```python
from build123d import *

# Parameters (mm, degrees)
SKETCH2_R           = 12
SKETCH2_R_2         = 2.2
SKETCH2_R_3         = 2.7
BOSS_EXTRUDE1_DEPTH = 5
SKETCH2_4_R         = 4.5
BOSS_EXTRUDE2_DEPTH = 2
FILLET1_R           = 5
FILLET2_R           = 5
SKETCH3_R           = 4.7
SKETCH3_R_2         = 2.7
BOSS_EXTRUDE3_DEPTH = 1
FILLET4_R           = 1
SKETCH4_R           = 6.5
SKETCH4_R_2         = 4.5
BOSS_EXTRUDE5_DEPTH = 1
BOSS_EXTRUDE6_DEPTH = 3


with BuildPart() as part:
    # Sketch2 → Boss-Extrude1 (new body)
    with BuildSketch(Plane(origin=(0, 0, 0), x_dir=(1, 0, 0), z_dir=(0, 1, 0))):
        with BuildLine():
            Line((-32.658907628, 22.065310299), (-15.027926619, -31.62041432))
            Line((-15.027926619, -31.62041432), (-3.044319626, -14.687822099))
            ThreePointArc((-3.044319626, -14.687822099), (14.508216797, 3.809415358), (-9.86730521, 11.297623108))
            Line((-9.86730521, 11.297623108), (-32.658907628, 22.065310299))
        make_face()
        with Locations(Location((0, 0, 0), (0, 0, 270))):
            Circle(SKETCH2_R, mode=Mode.SUBTRACT)
        with Locations(Location((-13.044155697, -18.431125905, 0), (0, 0, 270))):
            Circle(SKETCH2_R_2, mode=Mode.SUBTRACT)
        with Locations(Location((-22.604306415, 10.679200882, 0), (0, 0, 270))):
            Circle(SKETCH2_R_3, mode=Mode.SUBTRACT)
    extrude(amount=BOSS_EXTRUDE1_DEPTH)

    # Sketch2<4> → Boss-Extrude2 (add)
    # profile 1 of 2: a face of its own
    with BuildSketch(Plane(origin=(0, 0, 0), x_dir=(1, 0, 0), z_dir=(0, 1, 0))):
        with BuildLine():
            Line((9.028311423, 2.370559296), (-1.105938309, -11.948928841))
            ThreePointArc((-1.105938309, -11.948928841), (8.084823445, -8.867673306), (12, 0))
            ThreePointArc((12, 0), (5.567714695, 10.630171827), (-6.833425512, 9.864293983))
            Line((-6.833425512, 9.864293983), (9.028311423, 2.370559296))
        make_face()
    # profile 2 of 2: a face of its own
    with BuildSketch(Plane(origin=(0, 0, 0), x_dir=(1, 0, 0), z_dir=(0, 1, 0))):
        with BuildLine():
            ThreePointArc((-6.833425512, 9.864293983), (-11.606573438, -3.047532287), (-1.105938309, -11.948928841))
            Line((-1.105938309, -11.948928841), (9.028311423, 2.370559296))
            Line((9.028311423, 2.370559296), (-6.833425512, 9.864293983))
        make_face()
        with Locations(Location((0, 0, 0), (0, 0, 270))):
            Circle(SKETCH2_4_R, mode=Mode.SUBTRACT)
    extrude(amount=BOSS_EXTRUDE2_DEPTH)

    # Fillet1
    fillet1_edges = [part.edges().sort_by_distance(p)[0] for p in [
        (-15.027926619, 2.5, 31.62041432),
        (-32.658907628, 2.5, -22.065310299),
    ]]
    fillet(fillet1_edges, radius=FILLET1_R)

    # Fillet2
    fillet2_edges = [part.edges().sort_by_distance(p)[0] for p in [
        (-9.86730521, 2.5, -11.297623108),
        (-3.044319626, 2.5, 14.687822099),
    ]]
    fillet(fillet2_edges, radius=FILLET2_R)

    # Sketch3 → Boss-Extrude3 (add)
    with BuildSketch(Plane(origin=(0, 5, 0), x_dir=(1, 0, 0), z_dir=(0, 1, 0))):
        with Locations(Location((-22.604306415, 10.679200882, 0), (0, 0, 270))):
            Circle(SKETCH3_R)
        with Locations(Location((-22.604306415, 10.679200882, 0), (0, 0, 270))):
            Circle(SKETCH3_R_2, mode=Mode.SUBTRACT)
    extrude(amount=BOSS_EXTRUDE3_DEPTH)

    # Fillet4
    fillet4_edges = [part.edges().sort_by_distance(p)[0] for p in [
        (-22.604306415, 5, -15.379200882),
    ]]
    fillet(fillet4_edges, radius=FILLET4_R - 0.0001)  # a hair under: the kernel refuses the full size

    # Sketch4 → Boss-Extrude5 (add)
    with BuildSketch(Plane(origin=(0, 2, 0), x_dir=(1, 0, 0), z_dir=(0, 1, 0))):
        with Locations(Location((0, 0, 0), (0, 0, 270))):
            Circle(SKETCH4_R)
        with Locations(Location((0, 0, 0), (0, 0, 270))):
            Circle(SKETCH4_R_2, mode=Mode.SUBTRACT)
    extrude(amount=BOSS_EXTRUDE5_DEPTH)

    # Sketch4<4> → Boss-Extrude6 (add)
    with BuildSketch(Plane(origin=(0, 2, 0), x_dir=(1, 0, 0), z_dir=(0, 1, 0))):
        with BuildLine():
            ThreePointArc((1.596440485, 11.893333333), (0, 12), (-1.596440485, 11.893333333))
            ThreePointArc((-1.596440485, 11.893333333), (0, 10.4), (1.596440485, 11.893333333))
        make_face()
        with BuildLine():
            ThreePointArc((9.50170856, -7.329224682), (10.392304845, -6), (11.098149045, -4.564108651))
            ThreePointArc((11.098149045, -4.564108651), (9.006664199, -5.2), (9.50170856, -7.329224682))
        make_face()
        with BuildLine():
            ThreePointArc((-9.50170856, -7.329224682), (-9.006664199, -5.2), (-11.098149045, -4.564108651))
            ThreePointArc((-11.098149045, -4.564108651), (-10.392304845, -6), (-9.50170856, -7.329224682))
        make_face()
    extrude(amount=BOSS_EXTRUDE6_DEPTH)


solid = part.part
```
The listing builds one solid part. Answer for the finished solid, in the listing's coordinates (mm). A direction names the side the tool comes from. Give positions to 0.01 mm unless a question says otherwise; leave off trailing zeros. Write each loop counter-clockwise with the first axis right and the second up, starting at its lowest first coordinate (ties: lowest second). Pieces come first, ordered by that corner, then holes. Notation, with made-up numbers: (4, 37) -> (36, 37) arc R21 ccw to (36, 49) -> close; hole circle Ø10 at (20, 22.5). An arc over 180 degrees is marked (long way). Write item = value, one per line. Start each with the question number.
1) Straight lines are drawn through the part: line 1 along X through (y, z) = (2.1, 0); line 2 along Z through (x, y) = (2.5, 2.25); line 3 along X through (y, z) = (3.95, -10). For each, find the intervals that lie inside material, in ascending order.
2) The part is cut by section B-B, the plane z = 20. Determine the outline of the cut face in (x, y).
3) The part is cut by section C-C, the plane z = 10. Determine the outline of the cut face in (x, y), and give its area (3 significant figures).
4) The part is cut by section D-D, the plane y = 1. Determine the outline of the cut face in (x, z).
5) The part is cut by section A-A, the plane x = 0. Determine the outline of the cut face in (y, z), and give its area (3 significant figures).
6) Each of these flat-tipped pins is pushed along its axis until it touches: pin 1 (21.5 mm diameter, centred on x = -6.5, z = -5, fed in from +Y); pin 2 (3 mm diameter, centred on y = 2.5, z = 15, fed in from -X); pin 3 (14.5 mm diameter, centred on x = 0, z = 0, fed in from +Y). Where does it stop, or does it pass through?
7) Which of the six approach directions +Z, -Z, +X, -X, +Y, -Y give full straight-line access (tool end or side, diameter ignored) to faces 1 (the face through (5, 2, 5)), 2 (the face through (-19.927, 2.958, -11.031))?
8) Determine the mould class of faces 3 (the face through (-27.65, 2.54, -16.27)), 4 (the face through (-10.174, 2.535, -12.086)), 5 (the face through (-7.05, 2.46, 20.35)), 6 (the face through (4.42, 3, -1.54)) for opening direction X: +X half, -X half, draft (parallel to the pull), parting line (faces both ways), or undercut.
Solutions:
q1.line_1 = -25.41 to -12, -6.5 to -4.5, 4.5 to 6.5, 12 to 15
q1.line_2 = -14.79 to -11.74, -6 to -3.74, 3.74 to 6, 11.74 to 14.79
q1.line_3 = -28.7 to -25.22, -19.99 to -6.63, 6.63 to 11.18
q2.outline = (-18.84, 0) -> (-14.59, 0) -> (-14.59, 5) -> (-18.84, 5) -> close; (-11.5, 0) -> (-6.8, 0) -> (-6.8, 5) -> (-11.5, 5) -> close
q3.outline = (-22.13, 0) -> (11.18, 0) -> (11.18, 5) -> (6.63, 5) -> (6.63, 2) -> (-6.63, 2) -> (-6.63, 5) -> (-22.13, 5) -> close
q3.area = 127 mm²
q4.outline = (-29.03, -11.02) arc R5 ccw to (-22.14, -17.1) -> (-12.54, -12.56) arc R5 cw to (-7.8, -12.81) arc R15 ccw (long way) to (-0.5, 14.99) arc R5 cw to (-4.75, 17.1) -> (-9.29, 23.52) arc R5 ccw to (-18.13, 22.19) -> close; hole circle Ø5.4 at (-22.6, -10.68); hole circle Ø4.4 at (-13.04, 18.43); hole circle Ø9 at (0, 0)
q5.outline = (0, -15) -> (5, -15) -> (5, -10.4) -> (2, -10.4) -> (2, -6.5) -> (3, -6.5) -> (3, -4.5) -> (0, -4.5) -> close; (0, 4.5) -> (3, 4.5) -> (3, 6.5) -> (2, 6.5) -> (2, 12) -> (5, 12) -> (5, 15) -> (0, 15) -> close
q5.area = 68.8 mm²
q6.pin_1 = 5
q6.pin_2 = -20.98
q6.pin_3 = 3
q7.face_1 = +Y
q7.face_2 = +Y, -Y
q8.face_3 = parting line
q8.face_4 = undercut
q8.face_5 = +X half
q8.face_6 = undercut
